Geometry: final body of the model. Coordinates: model frame, mm. A direction names the side the tool comes from. Round coordinates to 2 decimals unless told otherwise and drop trailing zeros. Order: outer loops, then holes, each group sorted by start corner. A loop starts at its lowest first (then second) coordinate and runs counter-clockwise, first axis right, second up. Notation, with made-up numbers: (-9, 58) -> (45, 58) arc R29 cw to (45, 83) -> close; hole circle Ø7 at (7, 34.5). An arc over 180 degrees is marked (long way). Put each result on its own line as item: value.
```python
from build123d import *

# Parameters (mm, degrees)
F0_W         = 48
F0_H         = 50
F1_DEPTH     = 2
F3_DEPTH     = 2
F4_W         = 20
F4_H         = 5
F5_DEPTH     = 25
F6_T1_DEPTH  = 4.6464466094
F6_T3_DEPTH  = 4.6464466094
F6_T5_DEPTH  = 4.6464466094
F6_T7_DEPTH  = 5.5355339059
F6_T9_DEPTH  = 5.5355339059
F6_T11_DEPTH = 4.6464466094


# Not quite as in the source:
# - a fillet or chamfer that OpenCascade refuses, or shapes differently, is made with other operations: its cross-section is extruded or revolved along the edge and cut away or added
# - a feature names something its author has since deleted; it is built from what else it names


with BuildPart() as f1:
    # F0 (on Top) → F1 (new body)
    with BuildSketch(Plane.XY):
        with Locations((24, -25)):
            Rectangle(F0_W, F0_H)
    extrude(amount=F1_DEPTH)

    # F2 (on face) → F3 (join)
    with BuildSketch(Plane.XY.offset(2)):
        Polygon((1.75, -1.75), (1.75, -3.8964466094), (3.8964466094, -1.75), align=None)
        Polygon((44.1035533906, -1.75), (46.25, -3.8964466094), (46.25, -1.75), align=None)
        Polygon((46.25, -48.25), (46.25, -46.1035533906), (44.1035533906, -48.25), align=None)
        Polygon((3.8964466094, -48.25), (1.75, -46.1035533906), (1.75, -48.25), align=None)
        Polygon((3.8964466094, -46.1035533906), (1.75, -46.1035533906), (3.8964466094, -48.25), align=None)
        Polygon((44.1035533906, -48.25), (46.25, -46.1035533906), (44.1035533906, -46.1035533906), align=None)
    extrude(amount=F3_DEPTH)

    # F4 (on face) → F5 (cut)
    with BuildSketch(Plane.XY.offset(2)):
        with Locations((24, -45.5)):
            Rectangle(F4_W, F4_H)
    extrude(amount=-F5_DEPTH, mode=Mode.SUBTRACT)

    # F6: fillet of radius 0.5 on 14 edges, made by hand

    # F6_s2 → F6_t1 (cut)
    with BuildSketch(Plane.XZ.offset(44.8535533906)):
        with BuildLine():
            add(Edge.make_bspline(
                [(1.75, 3.5), (1.75, 4), (2.25, 4)],
                knots=[0, 0, 0, 1, 1, 1], degree=2, weights=[1, 1, 1]))
            Line((2.25, 4), (1.75, 4))
            Line((1.75, 4), (1.75, 3.5))
        make_face()
        with BuildLine():
            add(Edge.make_bspline(
                [(3.8964466094, 3.5), (3.8964466094, 4), (3.3964466094, 4)],
                knots=[0, 0, 0, 1, 1, 1], degree=2, weights=[1, 1, 1]))
            Line((3.3964466094, 4), (3.8964466094, 4))
            Line((3.8964466094, 4), (3.8964466094, 3.5))
        make_face()
        with BuildLine():
            add(Edge.make_bspline(
                [(46.25, 3.5), (46.25, 4), (45.75, 4)],
                knots=[0, 0, 0, 1, 1, 1], degree=2, weights=[1, 1, 1]))
            Line((45.75, 4), (46.25, 4))
            Line((46.25, 4), (46.25, 3.5))
        make_face()
        with BuildLine():
            add(Edge.make_bspline(
                [(44.1035533906, 3.5), (44.1035533906, 4), (44.6035533906, 4)],
                knots=[0, 0, 0, 1, 1, 1], degree=2, weights=[1, 1, 1]))
            Line((44.6035533906, 4), (44.1035533906, 4))
            Line((44.1035533906, 4), (44.1035533906, 3.5))
        make_face()
    extrude(amount=F6_T1_DEPTH, mode=Mode.SUBTRACT)

    # F6_s4 → F6_t3 (cut)
    with BuildSketch(Plane.YZ.offset(0.5)):
        with BuildLine():
            add(Edge.make_bspline(
                [(-48.25, 3.5), (-48.25, 4), (-47.75, 4)],
                knots=[0, 0, 0, 1, 1, 1], degree=2, weights=[1, 1, 1]))
            Line((-47.75, 4), (-48.25, 4))
            Line((-48.25, 4), (-48.25, 3.5))
        make_face()
        with BuildLine():
            add(Edge.make_bspline(
                [(-46.1035533906, 3.5), (-46.1035533906, 4), (-46.6035533906, 4)],
                knots=[0, 0, 0, 1, 1, 1], degree=2, weights=[1, 1, 1]))
            Line((-46.6035533906, 4), (-46.1035533906, 4))
            Line((-46.1035533906, 4), (-46.1035533906, 3.5))
        make_face()
        with BuildLine():
            add(Edge.make_bspline(
                [(-1.75, 3.5), (-1.75, 4), (-2.25, 4)],
                knots=[0, 0, 0, 1, 1, 1], degree=2, weights=[1, 1, 1]))
            Line((-2.25, 4), (-1.75, 4))
            Line((-1.75, 4), (-1.75, 3.5))
        make_face()
    extrude(amount=F6_T3_DEPTH, mode=Mode.SUBTRACT)

    # F6_s6 → F6_t5 (cut)
    with BuildSketch(Plane.XZ.offset(0.5)):
        with BuildLine():
            add(Edge.make_bspline(
                [(1.75, 3.5), (1.75, 4), (2.25, 4)],
                knots=[0, 0, 0, 1, 1, 1], degree=2, weights=[1, 1, 1]))
            Line((2.25, 4), (1.75, 4))
            Line((1.75, 4), (1.75, 3.5))
        make_face()
        with BuildLine():
            add(Edge.make_bspline(
                [(46.25, 3.5), (46.25, 4), (45.75, 4)],
                knots=[0, 0, 0, 1, 1, 1], degree=2, weights=[1, 1, 1]))
            Line((45.75, 4), (46.25, 4))
            Line((46.25, 4), (46.25, 3.5))
        make_face()
    extrude(amount=F6_T5_DEPTH, mode=Mode.SUBTRACT)

    # F6_s8 → F6_t7 (cut)
    with BuildSketch(Plane(origin=(-1.9571067812, -1.9571067812, 0), x_dir=(0, 0, 1), z_dir=(0.7071067812, 0.7071067812, 0))):
        with BuildLine():
            add(Edge.make_bspline(
                [(3.5, 3.9926406871), (4, 3.9926406871), (4, 3.4926406871)],
                knots=[0, 0, 0, 1, 1, 1], degree=2, weights=[1, 1, 1]))
            Line((4, 3.4926406871), (4, 3.9926406871))
            Line((4, 3.9926406871), (3.5, 3.9926406871))
        make_face()
    extrude(amount=F6_T7_DEPTH, mode=Mode.SUBTRACT)

    # F6_s10 → F6_t9 (cut)
    with BuildSketch(Plane(origin=(22.0428932188, -22.0428932188, 0), x_dir=(0, 0, 1), z_dir=(0.7071067812, -0.7071067812, 0))):
        with BuildLine():
            add(Edge.make_bspline(
                [(3.5, -29.9484848098), (4, -29.9484848098), (4, -30.4484848098)],
                knots=[0, 0, 0, 1, 1, 1], degree=2, weights=[1, 1, 1]))
            Line((4, -30.4484848098), (4, -29.9484848098))
            Line((4, -29.9484848098), (3.5, -29.9484848098))
        make_face()
    extrude(amount=F6_T9_DEPTH, mode=Mode.SUBTRACT)

    # F6_s12 → F6_t11 (cut)
    with BuildSketch(Plane.YZ.offset(42.8535533906)):
        with BuildLine():
            add(Edge.make_bspline(
                [(-1.75, 3.5), (-1.75, 4), (-2.25, 4)],
                knots=[0, 0, 0, 1, 1, 1], degree=2, weights=[1, 1, 1]))
            Line((-2.25, 4), (-1.75, 4))
            Line((-1.75, 4), (-1.75, 3.5))
        make_face()
        with BuildLine():
            add(Edge.make_bspline(
                [(-46.1035533906, 3.5), (-46.1035533906, 4), (-46.6035533906, 4)],
                knots=[0, 0, 0, 1, 1, 1], degree=2, weights=[1, 1, 1]))
            Line((-46.6035533906, 4), (-46.1035533906, 4))
            Line((-46.1035533906, 4), (-46.1035533906, 3.5))
        make_face()
        with BuildLine():
            add(Edge.make_bspline(
                [(-48.25, 3.5), (-48.25, 4), (-47.75, 4)],
                knots=[0, 0, 0, 1, 1, 1], degree=2, weights=[1, 1, 1]))
            Line((-47.75, 4), (-48.25, 4))
            Line((-48.25, 4), (-48.25, 3.5))
        make_face()
    extrude(amount=F6_T11_DEPTH, mode=Mode.SUBTRACT)


solid = f1.part
```
1. Cut plane B-B on x = 24. Return loops of the section in (y, z), and give its area (3 significant figures).
Ans:
outline: (-50, 0) -> (-48, 0) -> (-48, 2) -> (-50, 2) -> close; (-43, 0) -> (0, 0) -> (0, 2) -> (-43, 2) -> close
area: 90.0 mm²
2. Cut plane A-A on z = 2.65. Return loops of the section in (x, y).
Ans:
outline: (1.75, -48.25) -> (3.9, -48.25) -> (3.9, -46.1) -> (1.75, -46.1) -> close; (1.75, -3.9) -> (3.9, -1.75) -> (1.75, -1.75) -> close; (44.1, -48.25) -> (46.25, -48.25) -> (46.25, -46.1) -> (44.1, -46.1) -> close; (44.1, -1.75) -> (46.25, -3.9) -> (46.25, -1.75) -> close
3. Cut plane D-D on x = 5. Return loops of the section in (y, z).
Ans:
outline: (-50, 0) -> (0, 0) -> (0, 2) -> (-50, 2) -> close
4. Material intervals for probe 1 along Y at (x, z) = (25, 0.65); probe 2 along X at (y, z) = (-46.5, 0.8); probe 3 along Z at (x, y) = (24, -33), sorted ascending.
Ans:
probe 1: -50 to -48, -43 to 0
probe 2: 0 to 14, 34 to 48
probe 3: 0 to 2
5. Cut plane C-C on y = -14. Return loops of the section in (x, z).
Ans:
outline: (0, 0) -> (48, 0) -> (48, 2) -> (0, 2) -> close
6. Set-up query: faces 1 (the face through (2.808, -2.838, 2.74)), 2 (the face through (1.75, -3, 3)), 3 (the face through (3, -48.25, 3)). Return all of +Z, -Z, +X, -X, +Y, -Y with unobstructed straight access to the full face (end or side cutting, diameter ignored); none if empty.
Ans:
face 1: +Z
face 2: +Z, -X, +Y, -Y
face 3: +Z, +X, -X, -Y
7. Contact query for flat-ended pins moving along their axis: P1, Ø5, axis at x = 10, y = -23, coming from the +Z side; P2, Ø0.8, axis at x = 45.5, z = 3, coming from the +Y side; P3, Ø0.8, axis at x = 45.5, z = 3, coming from the -Y side. Output: stop coordinate, or through.
Ans:
P1: z = 2
P2: y = -1.75
P3: y = -48.25
8. Draft query along X for faces 4 (the face through (45, -46.104, 3)), 5 (the face through (14, -46, 1)), 6 (the face through (46.25, -47, 3)), 7 (the face through (45.162, -2.808, 2.74)). Return one class per face: +X half, -X half, draft (parallel to the pull), parting line (faces both ways), or undercut.
Ans:
face 4: draft
face 5: undercut
face 6: +X half
face 7: undercut
